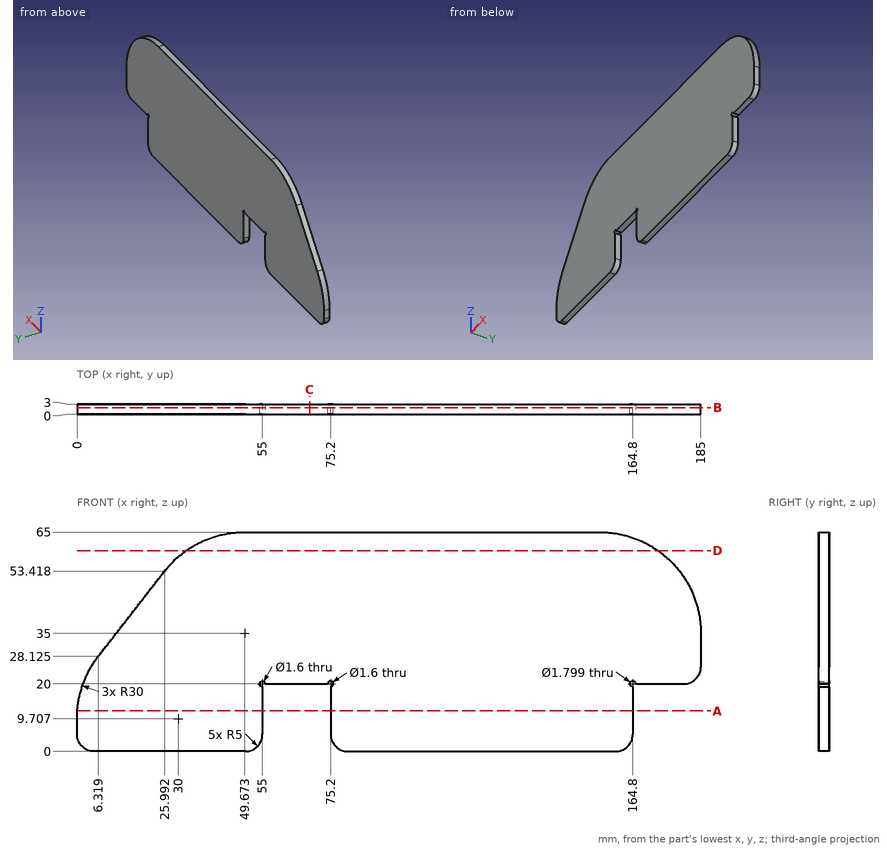
Job drawing, mm, ordinate dimensions from the low corner. One solid piece. Round coordinates to 2 decimals unless told otherwise and drop trailing zeros. Write each loop counter-clockwise with the first axis right and the second up, starting at its lowest first coordinate (ties: lowest second). Pieces come first, ordered by that corner, then holes. Notation, with made-up numbers: M 70.5,24.5 L 111.5,24.5 A8 cw 111.5,28.5 Z; hole C 21,36.5 d2. An arc over 180 degrees is marked long. Return JSON: item names as keys, results as strings. Group by question number.
(1) Saw through at A-A on z = 12. Write the cut outline in (x, y).
(2) Pin check, flat tips, straight feed: pin 1 Ø0.9 at (y, z) = (2, 12.5) entering from +X; pin 2 Ø1 at (y, z) = (1.5, 44) entering from +X; pin 3 Ø1.6 at (x, z) = (164.8, 20) entering from -Y; pin 4 Ø2 at (x, z) = (139.5, 54) entering from -Y. Stop position of each tip, or through.
(3) Saw through at C-C on x = 69. Write the cut outline in (y, z), then the cut area to 3 significant figures.
(4) Saw through at D-D on z = 59.5. Write the cut outline in (x, y), then the cut area to 3 significant figures.
(5) Drill centre lines: probe 1 along X at (y, z) = (1.15, 10); probe 2 along Z at (x, y) = (58, 1.85); probe 3 along X at (y, z) = (1.55, 45) (1 decimal). Where is each one in solid material? Low to high.
(6) Saw through at B-B on y = 1.95. Write the cut outline in (x, z) (1 decimal), then the cut area to 3 significant figures.
Returned:
{
 "1": {"outline": "M 0.09,0 L 55,0 L 55,3 L 0.09,3 Z; M 75.2,0 L 164.8,0 L 164.8,3 L 75.2,3 Z"},
 "2": {"pin 1": "x = 164.8", "pin 2": "x = 183.77", "pin 3": "through", "pin 4": "y = 0"},
 "3": {"outline": "M 0,20 L 3,20 L 3,65 L 0,65 Z", "area": "135 mm²"},
 "4": {"outline": "M 32.36,0 L 172.31,0 L 172.31,3 L 32.36,3 Z", "area": "420 mm²"},
 "5": {"probe 1": "0 to 55, 75.2 to 164.8", "probe 2": "20 to 65", "probe 3": "19.4 to 183.3"},
 "6": {"outline": "M 0,5 A5 ccw 5,0 L 50,0 A5 ccw 55,5 L 55,19.2 A0.8 cw long 55.8,20 L 74.4,20 A0.8 cw long 75.2,19.2 L 75.2,5 A5 ccw 80.2,0 L 159.8,0 A5 ccw 164.8,5 L 164.8,19.1 A0.9 cw long 165.7,20 L 180,20 A5 ccw 185,25 L 185,35 A30 ccw 155,65 L 49.7,65 A30 ccw 26,53.4 L 6.3,28.1 A30 ccw 0,9.7 Z", "area": "10,200 mm²"}
}
